For this review, use the dimensioned drawing (mm, ordinates from the lowest corner) and the shaded views. A direction names the side the tool comes from. Coordinates: 2 decimals unless noted, no trailing zeros. Loops run counter-clockwise (first coordinate to the right, second up) from the corner with the lowest first, then second, coordinate; pieces in that order, holes last. Notation, with made-up numbers: M 27.25,69 L 71.25,69 A36 ccw 71.25,103 Z; hole C 23,-16.5 d9. An arc over 180 degrees is marked long. One line per item, written item: value.
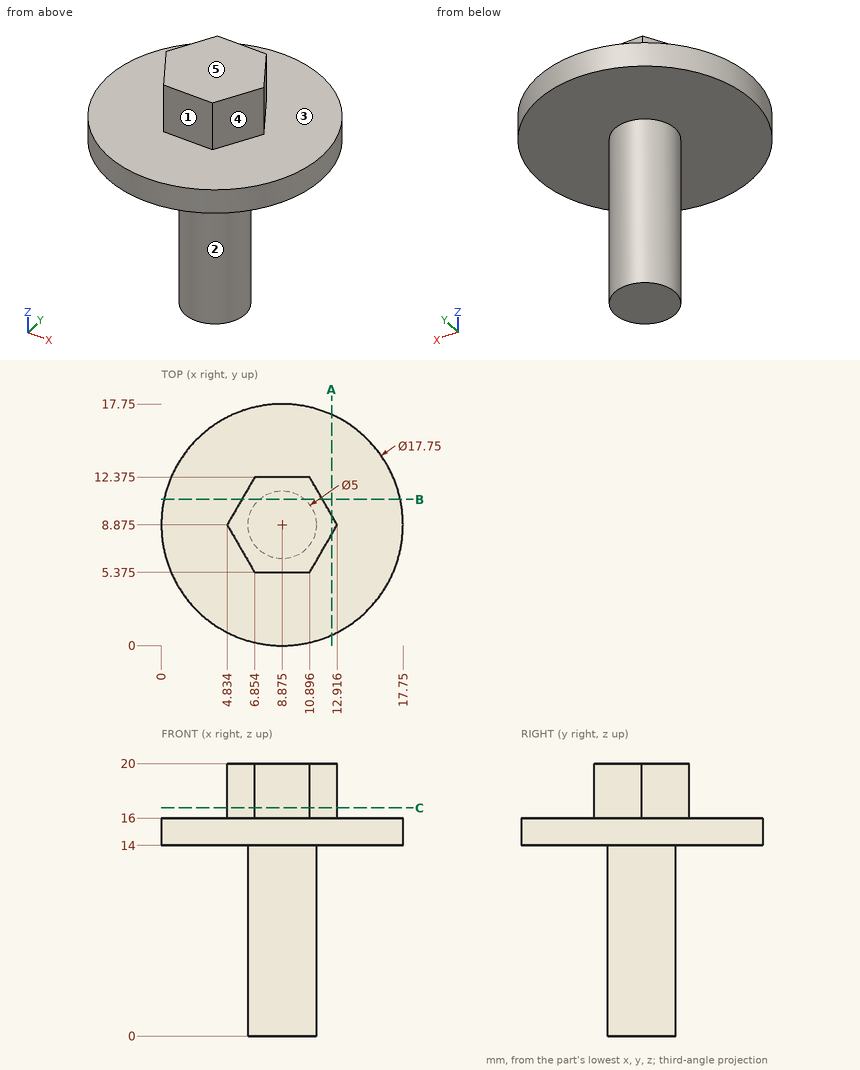
(1) Insertion check: pin 1 (5 mm diameter, centred on y = 13.5, z = 9, fed in from -X); pin 2 (5 mm diameter, centred on y = 5.5, z = 16, fed in from -X); pin 3 (2 mm diameter, centred on x = 7.5, z = 11.5, fed in from +Y); pin 4 (4 mm diameter, centred on y = 13.5, z = 8, fed in from -X). Each pin has a flat end and moves straight along its axis. Give the tip position at first contact, or say it passes through.
Reply:
pin 1: stops at x = 7.56
pin 2: stops at x = 0.04
pin 3: stops at y = 11.35
pin 4: passes through
(2) We need section B-B on y = 10.75. State the section outline as (x, z) points.
Reply:
outline: M 0.2,14 L 7.22,14 L 7.22,0 L 10.53,0 L 10.53,14 L 17.55,14 L 17.55,16 L 11.83,16 L 11.83,20 L 5.92,20 L 5.92,16 L 0.2,16 Z
(3) We need section A-A on x = 12.5. State the section outline as (y, z) points.
Reply:
outline: M 0.77,14 L 16.98,14 L 16.98,16 L 9.6,16 L 9.6,20 L 8.15,20 L 8.15,16 L 0.77,16 Z
(4) We need section C-C on z = 16.75. State the section outline as (x, y) points (1 decimal).
Reply:
outline: M 4.8,8.9 L 6.9,5.4 L 10.9,5.4 L 12.9,8.9 L 10.9,12.4 L 6.9,12.4 Z
(5) Tool access review of the marked faces 1, 2, 3, 4 and 5: name each direction out of +Z, -Z, +X, -X, +Y, -Y from which nothing blocks a thin tool from reaching the whole face with its end or side.
Reply:
face 1: +Z, +X, -X, -Y
face 2: -Z
face 3: +Z
face 4: +Z, +X, -Y
face 5: +Z, +X, -X, +Y, -Y
(6) To check wall thickness, follow line 1 along Z through (x, y) = (1, 5.5); line 2 along Z through (x, y) = (6.25, 7); line 3 along X through (y, z) = (7, 11.5). State the ranges of each line that lie inside material, in increasing order. Write a range as [from, to].
Reply:
line 1: z = [14, 16]
line 2: z = [14, 20]
line 3: x = [7.22, 10.53]
